For this review, take the finished solid that the model builds, in its own axes (mm). Face numbers are marked on the shaded views. A direction names the side the tool comes from. Coordinates: 2 decimals unless noted, no trailing zeros. Loops run counter-clockwise (first coordinate to the right, second up) from the corner with the lowest first, then second, coordinate; pieces in that order, holes last. Notation, with made-up numbers: (78.25, 77.25) -> (132.25, 77.25) arc R27 cw to (132.25, 94.25) -> close; hole circle Ø5 at (32, 24.25). An arc over 180 degrees is marked (long way). Use a Markdown table: item, result.
from build123d import *

# Parameters (mm, degrees)
SKETCH1_R           = 1.55
SKETCH1_R_2         = 4.25
SKETCH1_R_3         = 1.1
BOSS_EXTRUDE1_DEPTH = 5
CUT_EXTRUDE2_DEPTH  = 2
SKETCH4_R           = 1.75
CUT_EXTRUDE3_DEPTH  = 2.25
CHAFL_N1_SIZE       = 0.75


with BuildPart() as part:
    # Sketch1 → Boss-Extrude1 (new body)
    with BuildSketch(Plane.XY):
        with BuildLine():
            Line((-23.020815218, 6.216096398), (-25.999136894, -18.423903602))
            ThreePointArc((-25.999136894, -18.423903602), (-15.078624085, -30.743903602), (-4.158111277, -18.423903602))
            Line((-4.158111277, -18.423903602), (-7.136432952, 6.216096398))
            ThreePointArc((-7.136432952, 6.216096398), (-15.078624085, 13.256096398), (-23.020815218, 6.216096398))
        make_face()
        with Locations((-15.078624085, 5.256096398)):
            Circle(SKETCH1_R, mode=Mode.SUBTRACT)
        with Locations((-15.078624085, -19.743903602)):
            Circle(SKETCH1_R_2, mode=Mode.SUBTRACT)
        with Locations((-7.078624085, -19.743903602)):
            Circle(SKETCH1_R_3, mode=Mode.SUBTRACT)
        with Locations((-9.421769836, -25.400757851)):
            Circle(SKETCH1_R_3, mode=Mode.SUBTRACT)
        with Locations((-15.078624085, -27.743903602)):
            Circle(SKETCH1_R_3, mode=Mode.SUBTRACT)
        with Locations((-20.735478335, -25.400757851)):
            Circle(SKETCH1_R_3, mode=Mode.SUBTRACT)
        with Locations((-23.078624085, -19.743903602)):
            Circle(SKETCH1_R_3, mode=Mode.SUBTRACT)
        with Locations((-20.735478335, -14.087049352)):
            Circle(SKETCH1_R_3, mode=Mode.SUBTRACT)
        with Locations((-15.078624085, -11.743903602)):
            Circle(SKETCH1_R_3, mode=Mode.SUBTRACT)
        with Locations((-9.421769836, -14.087049352)):
            Circle(SKETCH1_R_3, mode=Mode.SUBTRACT)
    extrude(amount=BOSS_EXTRUDE1_DEPTH)

    # Sketch3 → Cut-Extrude2 (cut)
    with BuildSketch(Plane.XY):
        Polygon((-13.490910845, 2.506096398), (-11.903197604, 5.256096398), (-13.490910845, 8.006096398), (-16.666337325, 8.006096398), (-18.254050566, 5.256096398), (-16.666337325, 2.506096398), align=None)
    extrude(amount=CUT_EXTRUDE2_DEPTH, mode=Mode.SUBTRACT)

    # Sketch4 → Cut-Extrude3 (cut)
    with BuildSketch(Plane(origin=(0, 0, 0), x_dir=(-1, 0, 0), z_dir=(0, 0, -1))):
        with Locations((23.078624085, -19.743903602)):
            Circle(SKETCH4_R)
        with Locations((20.735478335, -25.400757851)):
            Circle(SKETCH4_R)
        with Locations((15.078624085, -27.743903602)):
            Circle(SKETCH4_R)
        with Locations((9.421769836, -25.400757851)):
            Circle(SKETCH4_R)
        with Locations((7.078624085, -19.743903602)):
            Circle(SKETCH4_R)
        with Locations((9.421769836, -14.087049352)):
            Circle(SKETCH4_R)
        with Locations((15.078624085, -11.743903602)):
            Circle(SKETCH4_R)
        with Locations((20.735478335, -14.087049352)):
            Circle(SKETCH4_R)
    extrude(amount=-CUT_EXTRUDE3_DEPTH, mode=Mode.SUBTRACT)

    # Chaflán1
    chafl_n1_edges = [part.edges().sort_by_distance(p)[0] for p in [
        (-5.647272114, -6.103903602, 0),
        (-15.078624085, -30.743903602, 0),
        (-24.509976056, -6.103903602, 0),
        (-15.078624085, 13.256096398, 0),
    ]]
    chamfer(chafl_n1_edges, length=CHAFL_N1_SIZE)


solid = part.part
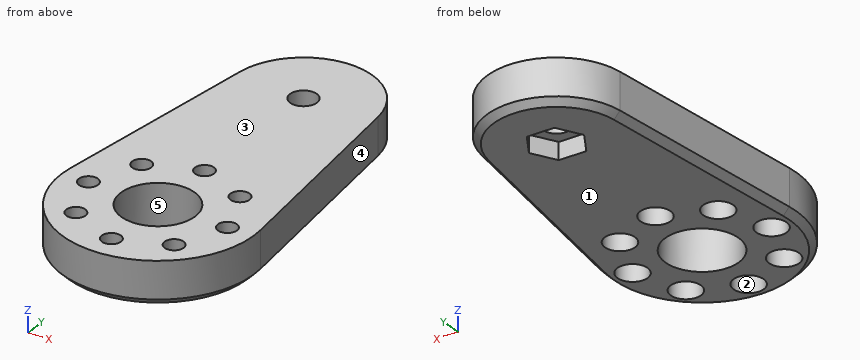
(1) Take a section at A-A on y = -17. Write out the cut boundary in (x, z).
Found:
| item | result |
|---|---|
| outline | (-25.83, 0.75) -> (-25.07, 0) -> (-18.32, 0) -> (-18.32, 5) -> (-25.83, 5) -> close; (-11.83, 0) -> (-5.09, 0) -> (-4.33, 0.75) -> (-4.33, 5) -> (-11.83, 5) -> close |
(2) Mouldability with a two-part tool opening along Y and no side actions: class the marked faces 3, 4 and 5 as pulls with the +Y half, pulls with the -Y half, needs draft (parallel to the pull), parting line crosses it, or undercut.
Found:
| item | result |
|---|---|
| face 3 | needs draft |
| face 4 | pulls with the +Y half |
| face 5 | undercut |
(3) For pin 1 Ø1 at (x, z) = (-8.5, 1) entering from +Y; pin 2 Ø3 at (x, y) = (-7.08, -19.74) entering from -Z; pin 3 Ø1.5 at (y, z) = (-16.5, 2.5) entering from -X, all flat-tipped, find the tip position at first contact; note any pin that passes through.
Found:
| item | result |
|---|---|
| pin 1 | stops at y = 10.46 |
| pin 2 | stops at z = 2.25 |
| pin 3 | stops at x = -25.86 |
(4) Take a section at B-B on z = 4. State how many separate pieces and enclosed holes the cut face has, plus the area to 3 significant figures.
Found:
| item | result |
|---|---|
| separate pieces | 1 |
| enclosed holes | 10 |
| area | 674 mm^2 |
(5) For the marked faces 1 and 2, list the 3-axis set-ups (+Z, -Z, +X, -X, +Y, -Y) from which the entire face can be reached by the end or side of a thin tool; tool diameter is ignored.
Found:
| item | result |
|---|---|
| face 1 | -Z, +X, -X, +Y, -Y |
| face 2 | -Z |
(6) For line 1 along Y through (x, z) = (-21.25, 0.7); line 2 along X through (y, z) = (-25.5, 2.95); line 3 along X through (y, z) = (-19, 2.15), list the stretches that pass through material, from the lowest coordinate up.
Found:
| item | result |
|---|---|
| line 1 | y = -28.79 to -27.07, -23.73 to -15.76, -12.41 to 10.27 |
| line 2 | x = -24.45 to -21.83, -19.64 to -10.52, -8.33 to -5.7 |
| line 3 | x = -26.05 to -24.66, -21.49 to -19.26, -10.89 to -8.66, -5.49 to -4.1 |
(7) Take a section at D-D on y = 1.5. Write out the cut boundary in (x, z).
Found:
| item | result |
|---|---|
| outline | (-23.59, 0.75) -> (-22.84, 0) -> (-7.32, 0) -> (-6.57, 0.75) -> (-6.57, 5) -> (-23.59, 5) -> close |
